Can you work these out from the drawing? Everything is in mm from the part's minimum corner. A direction names the side the tool comes from. Coordinates: 2 decimals unless noted, no trailing zeros. Write each loop counter-clockwise with the first axis right and the second up, starting at its lowest first coordinate (ties: lowest second). Pieces come first, ordered by that corner, then holes. Notation, with made-up numbers: (71, 47.5) -> (103, 47.5) arc R26 cw to (103, 85.5) -> close; hole circle Ø5 at (-20.5, -19.75). An arc over 180 degrees is marked (long way). Use a Markdown table: item, result. Add a question column.
Item 1: If we mould it in two halves opening along Y, with no side actions, what happens to the marked faces 4, 5 and 6? For each: pulls with the +Y half, pulls with the -Y half, needs draft (parallel to the pull), parting line crosses it, or undercut.
Item 2: On a 3-axis mill with a long thin cutter (end or side, diameter ignored), from which of +Z, -Z, +X, -X, +Y, -Y can I reach the whole of each face in a straight line? I mean the marked faces 1, 2 and 3. Say none if no direction works.
Item 3: Imagine slicing it at C-C, the plane x = 2.25. Write out the boundary of the cut face in (y, z).
Item 4: If I drill on line 1 along Z through (x, y) = (8, 21); line 2 along Y through (x, z) = (14.05, 21), over which ranges is the centre line in solid material (lowest first)? Write a range as from..to.
Item 5: Will these pins go through, and if not, where does the flat tip stop? pin 1 Ø2 at (y, z) = (16, 31.5) entering from +X; pin 2 Ø2 at (y, z) = (12.5, 20) entering from -X; pin 3 Ø1.5 at (x, z) = (9, 15.5) entering from +Y.
Item 6: Imagine slicing it at A-A, the plane z = 21. Write out the boundary of the cut face in (x, y), and give its area (3 significant figures).
Item 7: Imagine slicing it at D-D, the plane y = 3.5. Write out the boundary of the cut face in (x, z), and give its area (3 significant figures).
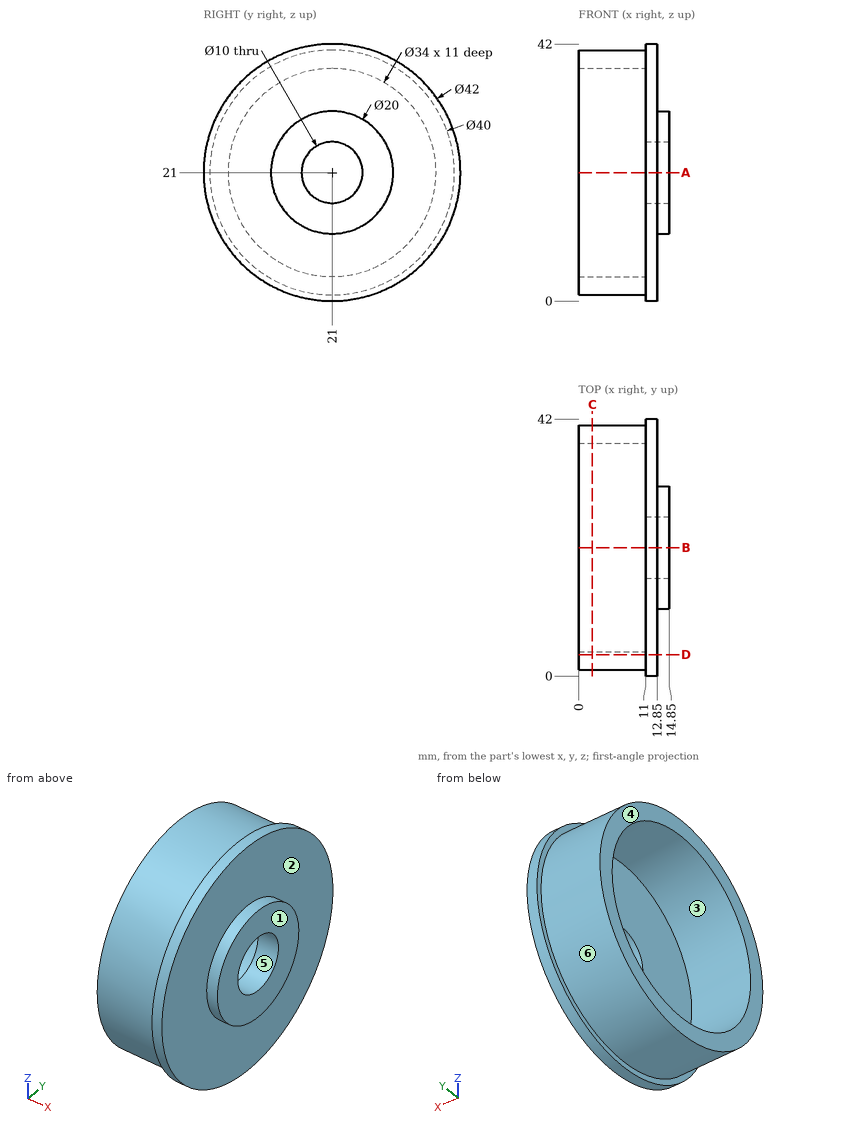
Ans:
| question | item | result |
|---|---|---|
| 1 | face 4 | needs draft |
| 1 | face 5 | undercut |
| 1 | face 6 | parting line crosses it |
| 2 | face 1 | +Z, -Z, +X, +Y, -Y |
| 2 | face 2 | +X |
| 2 | face 3 | -X |
| 3 | outline | circle Ø40 at (21, 21); hole circle Ø34 at (21, 21) |
| 4 | line 1 | z = 1..4, 38..41 |
| 4 | line 2 | y = 11..16, 26..31 |
| 5 | pin 1 | stops at x = 12.85 |
| 5 | pin 2 | stops at x = 11 |
| 5 | pin 3 | stops at y = 40.43 |
| 6 | outline | (0, 1) -> (11, 1) -> (11, 0) -> (12.85, 0) -> (12.85, 11) -> (14.85, 11) -> (14.85, 16) -> (11, 16) -> (11, 4) -> (0, 4) -> close; (0, 38) -> (11, 38) -> (11, 26) -> (14.85, 26) -> (14.85, 31) -> (12.85, 31) -> (12.85, 42) -> (11, 42) -> (11, 41) -> (0, 41) -> close |
| 6 | area | 145 mm^2 |
| 7 | outline | (0, 11.32) -> (11, 11.32) -> (11, 9.39) -> (12.85, 9.39) -> (12.85, 32.61) -> (11, 32.61) -> (11, 30.68) -> (0, 30.68) -> close |
| 7 | area | 256 mm^2 |
